Geometry check sheet. Reference: the model listing, model coordinates, mm. A direction names the side the tool comes from. Round coordinates to 2 decimals unless told otherwise and drop trailing zeros. Write each loop counter-clockwise with the first axis right and the second up, starting at its lowest first coordinate (ties: lowest second). Pieces come first, ordered by that corner, then holes. Notation, with made-up numbers: (68.5, -1.5) - (94.5, -1.5) arc R8 ccw to (94.5, 3.5) - close; hole circle Ø4 at (-22.5, 79.25). An arc over 180 degrees is marked (long way). One line per question, with ' | ' between items. Start each with the question number.
from build123d import *

# Parameters (mm, degrees)
F0_R     = 10
F1_DEPTH = 10
F2_R     = 10
F2_R_2   = 4
F3_DEPTH = 5
F4_R     = 10
F5_DEPTH = 0.6


with BuildPart() as f1:
    # F0 (on Right) → F1 (new body)
    with BuildSketch(Plane.YZ):
        Circle(F0_R)
        Polygon((0, 7.2168783649), (6.25, 3.6084391824), (6.25, -3.6084391824), (0, -7.2168783649), (-6.25, -3.6084391824), (-6.25, 3.6084391824), align=None, mode=Mode.SUBTRACT)
    extrude(amount=F1_DEPTH)

    # F2 (on face) → F3 (join)
    with BuildSketch(Plane.YZ.offset(10)):
        Circle(F2_R)
        Polygon((-6.25, 3.6084391824), (0, 7.2168783649), (6.25, 3.6084391824), (6.25, -3.6084391824), (0, -7.2168783649), (-6.25, -3.6084391824), align=None, mode=Mode.SUBTRACT)
        Polygon((6.25, 3.6084391824), (0, 7.2168783649), (-6.25, 3.6084391824), (-6.25, -3.6084391824), (0, -7.2168783649), (6.25, -3.6084391824), align=None)
        Circle(F2_R_2, mode=Mode.SUBTRACT)
    extrude(amount=F3_DEPTH)

    # F4 (on face) → F5 (join)
    with BuildSketch(Plane.YZ.offset(15)):
        Circle(F4_R)
    extrude(amount=F5_DEPTH)

    # F6 (on Front) → F7 (revolve)
    with BuildSketch(Plane.XZ):
        with BuildLine():
            ThreePointArc((19.6760818362, -15.0644853711), (17.075219414, -8.2618948834), (15.6, -1.1300332496))
            Line((15.6, -1.1300332496), (15.6, -10))
            Line((15.6, -10), (19.6760818362, -15.0644853711))
        make_face()
    revolve(axis=Axis((11.1028458923, 0, 0), (1, 0, 0)))


solid = f1.part
Q1. Section check B-B, the plane x = 13. Record the cut outline in (y, z), then the cut area to 3 significant figures.
Q2. Thickness scan on line 1 (Z direction, x = 12, y = 0); line 2 (Z direction, x = 14.25, y = 2.5); line 3 (X direction, y = 12.5, z = 6.5). Record the ranges inside material, lowest first.
Q3. Set-up check for faces 1 (the flat face through (4.93, -3.169, 5.387)), 2 (the flat face through (15.6, 0, 0)): record each of +Z, -Z, +X, -X, +Y, -Y from which the full face is reachable in a straight line by a thin tool's end or side.
Q4. Section check A-A, the plane x = 2.75. Record the cut outline in (y, z), then the cut area to 3 significant figures.
Q5. Draft check along Z on faces 3 (the conical face through (15.855, -10.071, 2.236)), 4 (the flat face through (0, 7, 0)), 5 (the flat face through (4.93, -3.08, -5.44)). Enter one of: pulls with the +Z half, pulls with the -Z half, needs draft (parallel to the pull), parting line crosses it, or undercut.
Q6. Go/stop test with flat-tipped pins: P1, Ø5, axis at y = -8.5, z = 3, coming from the -X side; P2, Ø1, axis at x = 13.5, y = -3, coming from the +Z side; P3, Ø2, axis at x = 7, z = -1.5, coming from the -Y side; P4, Ø2.5, axis at y = 0, z = 0.5, coming from the +X side. Record where each tip stops, or that it passes through.
Result sheet:
1) outline: circle Ø20 at (0, 0); hole circle Ø8 at (0, 0) | area: 264 mm²
2) line 1: -10 to -4, 4 to 10 | line 2: -9.68 to -3.12, 3.12 to 9.68 | line 3: 18.89 to 19.22
3) face 1: -X | face 2: +X
4) outline: circle Ø20 at (0, 0); hole (-6.25, -3.61) - (0, -7.22) - (6.25, -3.61) - (6.25, 3.61) - (0, 7.22) - (-6.25, 3.61) - close | area: 179 mm²
5) face 3: parting line crosses it | face 4: needs draft | face 5: undercut
6) P1: x = 0 | P2: z = 9.68 | P3: y = -9.99 | P4: x = 15.68
